Geometry: final body of the model. Coordinates: model frame, mm. Face numbers are marked on the shaded views. A direction names the side the tool comes from. Coordinates: 2 decimals unless noted, no trailing zeros. Write each loop counter-clockwise with the first axis right and the second up, starting at its lowest first coordinate (ties: lowest second). Pieces come first, ordered by that corner, then holes. Notation, with made-up numbers: (86, 19.25) -> (113, 19.25) arc R22 ccw to (113, 35.25) -> close; hole circle Ø2 at (-35.75, -35.75). An arc over 180 degrees is marked (long way). One line per item, written item: value. Start each with the question number.
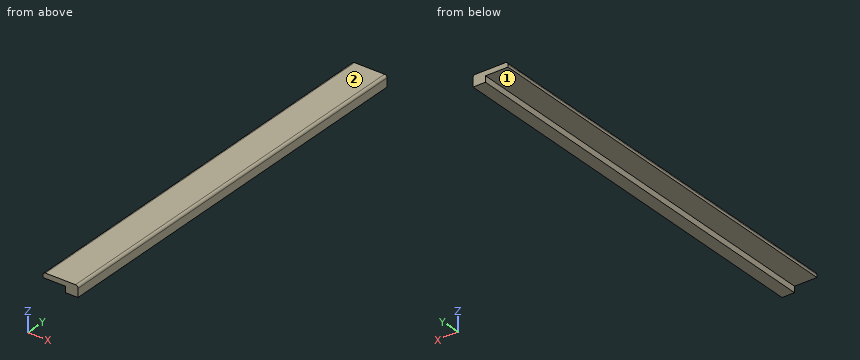
from build123d import *

# Parameters (mm, degrees)
F1_DEPTH = 820


with BuildPart() as f1:
    # F0 (on Front) → F1 (new body)
    with BuildSketch(Plane.XZ):
        with BuildLine():
            Line((0, 5), (0, 0))
            Line((0, 0), (45, 0))
            Line((45, 0), (45, -12))
            Line((45, -12), (70, -12))
            Line((70, -12), (70, 5))
            ThreePointArc((70, 5), (68.535534, 8.535534), (65, 10))
            Line((65, 10), (5, 10))
            ThreePointArc((5, 10), (1.464466, 8.535534), (0, 5))
        make_face()
    extrude(amount=F1_DEPTH)


solid = f1.part
Q1. Access query for the marked faces 1 and 2. Directions: +Z, -Z, +X, -X, +Y, -Y. A direction counts if a zero-diameter tool reaches every point of the face in a straight line with its end or side. Return the directions, or none.
Q2. Cut plane A-A on y = -86.5. Output: boundary loops of the cut face in (x, z).
Q3. Cut plane B-B on z = -4.25. Output: boundary loops of the cut face in (x, y), and give its area (3 significant figures).
Q4. Line query: L1, parallel to Z at x = 65.5, y = -127; L2, parallel to X at y = -415, z = -4.5; L3, parallel to Z at x = 7, y = -459. Output: solid intervals per line, ascending. Write a range as from..to.
Q5. First-contact query: P1, Ø8, axis at x = 55, z = 1, coming from the +Y side; P2, Ø3.5, axis at y = -489.5, z = -5.5, coming from the -X side. Flat tips, straight axial feed; report the tip coordinate or a pass-through.
Q6. Cut plane C-C on x = 23. Output: boundary loops of the cut face in (y, z).
Solution:
1. face 1: -Z, -X, +Y, -Y
1. face 2: +Z, +X, -X, +Y, -Y
2. outline: (0, 0) -> (45, 0) -> (45, -12) -> (70, -12) -> (70, 5) arc R5 ccw to (65, 10) -> (5, 10) arc R5 ccw to (0, 5) -> close
3. outline: (45, -820) -> (70, -820) -> (70, 0) -> (45, 0) -> close
3. area: 20,500 mm²
4. L1: -12..9.97
4. L2: 45..70
4. L3: 0..10
5. P1: y = 0
5. P2: x = 45
6. outline: (-820, 0) -> (0, 0) -> (0, 10) -> (-820, 10) -> close
